Work out the finished part from the listing and answer in its coordinate system (mm). A direction names the side the tool comes from. Coordinates: 2 decimals unless noted, no trailing zeros. Loops run counter-clockwise (first coordinate to the right, second up) from the corner with the lowest first, then second, coordinate; pieces in that order, holes last.
Autodesk Inventor part; units mm, degrees
ref_plane "YZ Plane" through (0, 0, 0) normal (1, 0, 0) x (0, 1, 0)
ref_plane "XZ Plane" through (0, 0, 0) normal (0, 1, 0) x (-1, 0, 0)
ref_plane "XY Plane" through (0, 0, 0) normal (0, 0, 1) x (1, 0, 0)
sketch "Sketch1" plane through (0, 0, 0) normal (0, 0, 1) x (1, 0, 0)
  circle A0 centre (0, 0) radius 53.5
  line L0 (38, -61) -> (-38, -61)
  line L1 (-40, -59) -> (-40, -35.5282)
  line L2 (40, -61) -> (-40, 61) construction
  line L3 (-40, -61) -> (40, 61) construction
  circle A1 centre (0, 27.5) radius 21
  line L4 (40, -35.5282) -> (40, -59)
  arc A2 (-40, -59) -> (-38, -61) centre (-38, -59) ccw
  arc A3 (38, -61) -> (40, -59) centre (38, -59) ccw
  dimension "d0" = 107
  dimension "d3" = 42
  dimension "d4" = 27.5
  dimension "d5" = 61
  dimension "d7" = 80
  dimension "d8" = 2
extrude "Extrusion1" add sketch "Sketch1" along normal blind 20
sketch "Sketch2" plane through (0, 0, 20) normal (0, 0, 1) x (1, 0, 0)
  line L0 (38, -61) -> (-38, -61)
  line L1 (-40, -59) -> (-40, -29.5)
  line L2 (-38, -27.5) -> (38, -27.5)
  line L3 (40, -29.5) -> (40, -59)
  arc A0 (-38, -27.5) -> (-40, -29.5) centre (-38, -29.5) ccw
  arc A1 (40, -29.5) -> (38, -27.5) centre (38, -29.5) ccw
  arc A2 (38, -61) -> (40, -59) centre (38, -59) ccw
  arc A3 (-40, -59) -> (-38, -61) centre (-38, -59) ccw
  point P0 (0, 0)
  point P1 (-40, -27.5)
  point P2 (-40, -61)
  point P3 (40, -27.5)
  dimension "d11" = 80
  dimension "d12" = 33.5
  dimension "d13" = 2
extrude "Extrusion2" add sketch "Sketch2" along normal blind 13
properties part number "ZWO-EFW-Mini" material "Steel"
1. Straight lines are drawn through the part: probe 1 along Y at (x, z) = (0, 6); probe 2 along X at (y, z) = (-31, 22); probe 3 along Z at (x, y) = (33, 30). For each, find the intervals that lie inside material, in ascending order.
2. Determine the mould class of faces 1 (the flat face through (1, -61, 16)), 2 (the cylindrical face through (9.69, 46.13, 9.86)), 3 (the flat face through (-1, -3, 0)) for opening direction Y: released by +Y, released by -Y, zero draft, split by the parting line, or undercut.
3. A cutting plane is placed at D-D, the plane y = 41. Give the vertices of the cut face in (x, z), then the cut area to 3 significant figures.
4. A cutting plane is placed at C-C, the plane z = 30. Give the vertices of the cut face in (x, y).
5. A cutting plane is placed at A-A, the plane x = 0. Give the vertices of the cut face in (y, z).
6. For faces 4 (the flat face through (-1, -44, 33)), 5 (the flat face through (-1, -27.5, 26)), determine the directions among +Z, -Z, +X, -X, +Y, -Y from which every point of the face is accessible in a straight line to the end or side of a thin tool.
7. A cutting plane is placed at B-B, the plane y = 27.5. Give the vertices of the cut face in (x, z), then the cut area to 3 significant figures.
8. Each of these flat-tipped pins is pushed along its axis until it touches: P1, Ø12, axis at y = -3.5, z = 18.5, coming from the -X side; P2, Ø10, axis at y = 3, z = 23.5, coming from the +X side; P3, Ø4, axis at y = 39.5, z = 18.5, coming from the -X side; P4, Ø25, axis at x = 0, y = 27.5, coming from the +Z side. Where does it stop, or does it pass through?
Answers below:
1. probe 1: y = -61 to 6.5, 48.5 to 53.5
1. probe 2: x = -40 to 40
1. probe 3: z = 0 to 20
2. face 1: released by -Y
2. face 2: undercut
2. face 3: zero draft
3. outline: (-34.37, 0) - (-16.09, 0) - (-16.09, 20) - (-34.37, 20) - close; (16.09, 0) - (34.37, 0) - (34.37, 20) - (16.09, 20) - close
3. area: 731 mm2
4. outline: (-40, -59) arc R2 ccw to (-38, -61) - (38, -61) arc R2 ccw to (40, -59) - (40, -29.5) arc R2 ccw to (38, -27.5) - (-38, -27.5) arc R2 ccw to (-40, -29.5) - close
5. outline: (-61, 0) - (6.5, 0) - (6.5, 20) - (-27.5, 20) - (-27.5, 33) - (-61, 33) - close; (48.5, 0) - (53.5, 0) - (53.5, 20) - (48.5, 20) - close
6. face 4: +Z, +X, -X, +Y, -Y
6. face 5: +Z, +X, -X, +Y
7. outline: (-45.89, 0) - (-21, 0) - (-21, 20) - (-45.89, 20) - close; (21, 0) - (45.89, 0) - (45.89, 20) - (21, 20) - close
7. area: 996 mm2
8. P1: stops at x = -53.5
8. P2: stops at x = 53.5
8. P3: stops at x = -38.16
8. P4: passes through
